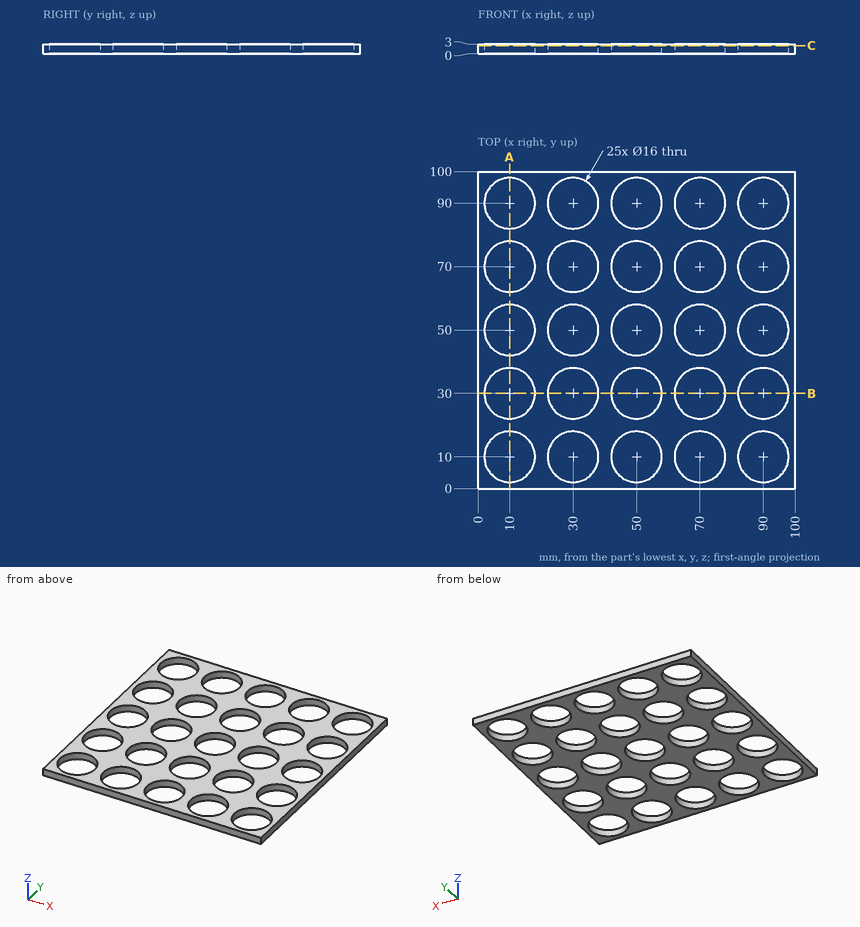
Answer from the drawing. Dimensions are ordinates in mm from the lowest x, y and z of the part. Coordinates: 2 decimals unless noted, no trailing zeros. Order: outer loops, then holes, each group sorted by start corner. A loop starts at its lowest first (then second) coordinate and runs counter-clockwise, first axis right, second up. Notation, with made-up numbers: M 12,-40 L 31,-40 A30 ccw 31,-13 Z; hole C -15.5,74 d9. An arc over 180 degrees is marked long. Put each result on its own line as item: value. Start each with the question number.
Item 1: Section A-A, the plane x = 10 is taken. Determine the outline of the cut face in (y, z).
Item 2: Consider probe 1 along Y at (x, z) = (50.5, 1.55); probe 2 along X at (y, z) = (87, 2.2); probe 3 along X at (y, z) = (86.5, 0.2). Determine where each line is inside the solid, lowest interval first. Write a range as [from, to].
Item 3: Section C-C, the plane z = 2.45 is taken. Count the separate pieces of the cut face and the enclosed holes in it, plus the area to 3 significant figures.
Computed:
1. outline: M 0,0 L 2,0 L 2,3 L 0,3 Z; M 18,0 L 22,0 L 22,3 L 18,3 Z; M 38,0 L 42,0 L 42,3 L 38,3 Z; M 58,0 L 62,0 L 62,3 L 58,3 Z; M 78,0 L 82,0 L 82,3 L 78,3 Z; M 98,0 L 100,0 L 100,3 L 98,3 Z
2. probe 1: y = [0, 2.02], [17.98, 22.02], [37.98, 42.02], [57.98, 62.02], [77.98, 82.02], [97.98, 100]
2. probe 2: x = [0, 2.58], [17.42, 22.58], [37.42, 42.58], [57.42, 62.58], [77.42, 82.58], [97.42, 100]
2. probe 3: x = [0, 2.81], [17.19, 22.81], [37.19, 42.81], [57.19, 62.81], [77.19, 82.81], [97.19, 100]
3. separate pieces: 1
3. enclosed holes: 25
3. area: 4,970 mm2
